```python
from build123d import *

# Parameters (mm, degrees)
F0_W     = 25
F0_H     = 40
F1_DEPTH = 4.9
F2_R     = 1.27
F3_W     = 2.54
F3_H     = 1.016
F4_DEPTH = 3


with BuildPart() as f1:
    # F0 (on Top) → F1 (new body)
    with BuildSketch(Plane.XY):
        Rectangle(F0_W, F0_H)
    extrude(amount=F1_DEPTH)

    # F2
    f2_edges = [f1.edges().sort_by_distance(p)[0] for p in [
        (-12.5, 0, 4.9),
        (12.5, 0, 4.9),
        (12.5, 0, 0),
        (-12.5, 0, 0),
    ]]
    fillet(f2_edges, radius=F2_R)

    # F3 (on face) → F4 (join)
    with BuildSketch(Plane.XZ.offset(20)):
        with Locations((6.785, 2.36)):
            Rectangle(F3_W, F3_H)
    extrude(amount=F4_DEPTH)


solid = f1.part
```
Can you work these out from the model? Positions are in its coordinate system, mm. A direction names the side the tool comes from. Coordinates: 2 decimals unless noted, no trailing zeros. Write each loop counter-clockwise with the first axis right and the second up, starting at its lowest first coordinate (ties: lowest second). Pieces come first, ordered by that corner, then holes. Notation, with made-up numbers: M 8.25,88 L 23.25,88 A25 cw 23.25,109 Z; hole C 4.25,75 d8. An arc over 180 degrees is marked long. Write item = value, one per line. Start each with the question number.
Q1. If we section it at A-A, the plane x = 2: Write out the boundary of the cut face in (y, z), then the cut area to 3 significant figures.
Q2. On a 3-axis mill with a long thin cutter (end or side, diameter ignored), from which of +Z, -Z, +X, -X, +Y, -Y can I reach the whole of each face in a straight line? I mean faces 1 (the face through (5.515, -21.5, 2.4)), 2 (the face through (8.055, -21.5, 2.4)), 3 (the face through (7, -21, 2.868)), 4 (the face through (7, -21, 1.852)). Say none if no direction works.
Q3. I'm going to push flat-ended pins straight in: pin 1 (2.5 mm diameter, centred on x = -5, z = 2, fed in from -Y); pin 2 (0.5 mm diameter, centred on y = -22, z = 2.5, fed in from +X) (3 decimals); pin 3 (0.8 mm diameter, centred on x = 6.5, y = -22, fed in from +Z). Where does each tip first touch, or does it pass through?
Q4. If I drill on L1, parallel to Y at x = 9.5, z = 1.2; L2, parallel to X at y = -2, z = 3.75; L3, parallel to X at y = -1.5, z = 4.2, over which ranges is the centre line in solid material (lowest first)? Write a range as [from, to].
Check sheet entries:
q1.outline = M -20,0 L 20,0 L 20,4.9 L -20,4.9 Z
q1.area = 196 mm²
q2.face_1 = +Z, -Z, -X, -Y
q2.face_2 = +Z, -Z, +X, -Y
q2.face_3 = +Z, +X, -X, -Y
q2.face_4 = -Z, +X, -X, -Y
q3.pin_1 = -20
q3.pin_2 = 8.055
q3.pin_3 = 2.87
q4.L1 = [-20, 20]
q4.L2 = [-12.49, 12.49]
q4.L3 = [-12.36, 12.36]
